Autodesk Inventor part; units mm, degrees
ref_plane "YZ Plane" through (0, 0, 0) normal (1, 0, 0) x (0, 1, 0)
ref_plane "XZ Plane" through (0, 0, 0) normal (0, 1, 0) x (-1, 0, 0)
ref_plane "XY Plane" through (0, 0, 0) normal (0, 0, 1) x (1, 0, 0)
sketch "Sketch1" plane through (0, 0, 0) normal (0, 0, 1) x (1, 0, 0)
  line L0 (0, 0) -> (0, 38.1)
  line L1 (0, 38.1) -> (38.1, 38.1)
  line L2 (38.1, 38.1) -> (38.1, 0)
  line L3 (38.1, 0) -> (0, 0)
  circle A0 centre (19.05, 19.05) radius 6.35
  circle A1 centre (3.175, 34.925) radius 2.3495
  circle A2 centre (34.925, 34.925) radius 2.3495
  circle A3 centre (3.175, 3.175) radius 2.3495
  circle A4 centre (34.925, 3.175) radius 2.3495
  dimension "d0" = 38.1
  dimension "d1" = 38.1
  dimension "d2" = 12.7
  dimension "d3" = 19.05
  dimension "d4" = 19.05
  dimension "d34" = 4.699
  dimension "d37" = 31.75
  dimension "d40" = 31.75
  dimension "d43" = 3.175
  dimension "d44" = 3.175
extrude "Extrusion1" add sketch "Sketch1" along normal blind 38.1
fillet "Fillet1" radius 3.175 4 edges at (38.1, 38.1, 19.05) (38.1, 0, 19.05) (0, 38.1, 19.05) (0, 0, 19.05)
sketch "Sketch2" plane through (0, 38.1, 0) normal (0, 1, 0) x (1, 0, 0)
  line L0 (0, 0) -> (38.1, 0)
  line L1 (0, 0) -> (0, -38.1)
  circle A0 centre (9.525, -3.81) radius 2.3495
  circle A1 centre (28.575, -3.81) radius 2.3495
  circle A2 centre (9.525, -30.48) radius 2.3495
  circle A3 centre (28.575, -30.48) radius 2.3495
  dimension "d8" = 4.699
  dimension "d11" = 19.05
  dimension "d14" = 26.67
  dimension "d17" = 3.81
  dimension "d18" = 9.525
extrude "Extrusion2" cut sketch "Sketch2" against normal blind 7.62
sketch "Sketch3" plane through (0, 0, 0) normal (0, -1, 0) x (1, 0, 0)
  line L0 (38.1, 0) -> (0, 0)
  line L1 (38.1, 0) -> (38.1, 38.1)
  circle A0 centre (28.575, 3.81) radius 2.3495
  circle A1 centre (9.525, 3.81) radius 2.3495
  circle A2 centre (28.575, 30.48) radius 2.3495
  circle A3 centre (9.525, 30.48) radius 2.3495
  dimension "d21" = 4.699
  dimension "d24" = 19.05
  dimension "d27" = 26.67
  dimension "d30" = 3.81
  dimension "d31" = 9.525
extrude "Extrusion3" cut sketch "Sketch3" against normal blind 7.62
properties part number "Base"
Work out the finished part from the listing and answer in its coordinate system (mm). A direction names the side the tool comes from. Coordinates: 2 decimals unless noted, no trailing zeros. Write each loop counter-clockwise with the first axis right and the second up, starting at its lowest first coordinate (ties: lowest second). Pieces come first, ordered by that corner, then holes.
Q1. Each of these flat-tipped pins is pushed along its axis until it touches: pin 1 Ø5 at (x, z) = (29.5, 5) entering from -Y; pin 2 Ø1.4 at (x, z) = (8.5, 3) entering from +Y; pin 3 Ø4 at (x, z) = (9.525, 30.48) entering from -Y. Where does it stop, or does it pass through?
Q2. A cutting plane is placed at A-A, the plane y = 19.05. Give the vertices of the cut face in (x, z), then the cut area to 3 significant figures.
Q3. Which of the six approach directions +Z, -Z, +X, -X, +Y, -Y give full straight-line access (tool end or side, diameter ignored) to faces 4 (the face through (9, 7.62, 4)), 5 (the face through (19, 28, 0)), 6 (the face through (29, 30.48, 4))?
Q4. Determine the mould class of faces 1 (the face through (0, 19, 19)), 2 (the face through (29, 7.62, 31)), 3 (the face through (37.166, 2.469, 18.783)) for opening direction Y: released by +Y, released by -Y, zero draft, split by the parting line, or undercut.
Q5. Find the intervals of material crossed by line 1 (Z direction, x = 28.5, y = 5); line 2 (Y direction, x = 3, z = 17.5); line 3 (Y direction, x = 36, z = 10), in increasing order.
Q6. A cutting plane is placed at D-D, the plane y = 4. Give the vertices of the cut face in (x, z) (1 decimal), then the cut area to 3 significant figures.
Q7. A cutting plane is placed at C-C, the plane z = 15.5. State how many separate pieces and enclosed holes the cut face has, then the cut area to 3 significant figures.
Findings below:
1. pin 1: stops at y = 0
1. pin 2: stops at y = 30.48
1. pin 3: stops at y = 7.62
2. outline: (0, 0) - (12.7, 0) - (12.7, 38.1) - (0, 38.1) - close; (25.4, 0) - (38.1, 0) - (38.1, 38.1) - (25.4, 38.1) - close
2. area: 968 mm2
3. face 4: -Y
3. face 5: -Z, +X, -X, +Y, -Y
3. face 6: +Y
4. face 1: zero draft
4. face 2: released by -Y
4. face 3: undercut
5. line 1: z = 0 to 1.46, 6.16 to 28.13, 32.83 to 38.1
5. line 2: y = 0 to 0.83, 5.52 to 32.58, 37.27 to 38.1
5. line 3: y = 0.19 to 1.09, 5.26 to 32.84, 37.01 to 37.91
6. outline: (0, 0) - (1, 0) - (1, 38.1) - (0, 38.1) - close; (5.4, 0) - (32.7, 0) - (32.7, 38.1) - (5.4, 38.1) - close; (37.1, 0) - (38.1, 0) - (38.1, 38.1) - (37.1, 38.1) - close; hole circle Ø4.7 at (9.5, 3.8); hole circle Ø4.7 at (9.5, 30.5); hole circle Ø4.7 at (28.6, 3.8); hole circle Ø4.7 at (28.6, 30.5)
6. area: 1,050 mm2
7. separate pieces: 1
7. enclosed holes: 5
7. area: 1,250 mm2
